The model under review builds one solid part; all positions refer to its coordinate system, in mm. Face numbers are marked on the shaded views. A direction names the side the tool comes from. Coordinates: 2 decimals unless noted, no trailing zeros. Order: outer loops, then holes, each group sorted by start corner. A loop starts at its lowest first (then second) coordinate and runs counter-clockwise, first axis right, second up. Notation, with made-up numbers: M -16,87.5 L 23,87.5 A29 cw 23,125.5 Z; hole C -5,46 d5. An arc over 180 degrees is marked long. One line per item, written item: value.
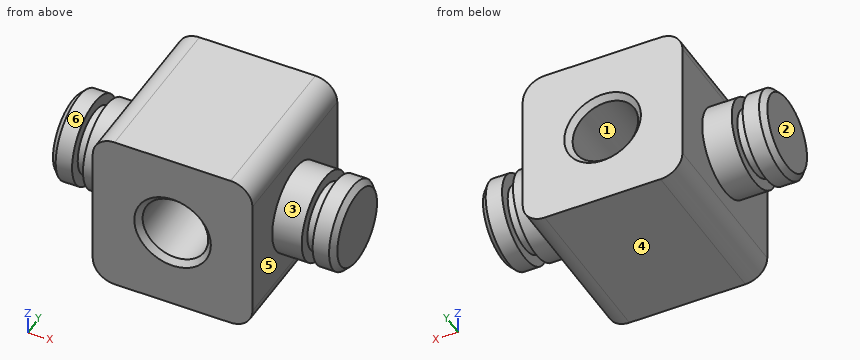
```python
from build123d import *

# Parameters (mm, degrees)
F2_DEPTH  = 381
F3_R      = 101.6
F4_DEPTH  = 68.58
F5_R      = 101.6
F6_DEPTH  = 68.58
F7_R      = 76.2
F8_DEPTH  = 508
F9_SIZE2  = 12.7
F9_SIZE   = 12.7
F11_R     = 76.2
F12_DEPTH = 25.4
F10_R     = 76.2
F13_DEPTH = 25.4
F14_R     = 101.6
F14_R_2   = 76.2
F15_DEPTH = 50.8
F16_R     = 101.6
F17_DEPTH = 50.8
F18_SIZE2 = 12.7
F18_SIZE  = 12.7


with BuildPart() as f2:
    # F1 (on Front) → F2 (new body)
    with BuildSketch(Plane.XZ):
        with BuildLine():
            ThreePointArc((-185.42, -139.7), (-170.541024, -175.621024), (-134.62, -190.5))
            Line((-134.62, -190.5), (134.62, -190.5))
            ThreePointArc((134.62, -190.5), (170.541024, -175.621024), (185.42, -139.7))
            Line((185.42, -139.7), (185.42, 139.7))
            ThreePointArc((185.42, 139.7), (170.541024, 175.621024), (134.62, 190.5))
            Line((134.62, 190.5), (-134.62, 190.5))
            ThreePointArc((-134.62, 190.5), (-170.541024, 175.621024), (-185.42, 139.7))
            Line((-185.42, 139.7), (-185.42, -139.7))
        make_face()
    extrude(amount=F2_DEPTH)

    # F3 (on face) → F4 (join)
    with BuildSketch(Plane.YZ.offset(185.42)):
        with Locations((-190.5, 0)):
            Circle(F3_R)
    extrude(amount=F4_DEPTH)

    # F5 (on face) → F6 (join)
    with BuildSketch(Plane(origin=(-185.42, 0, 0), x_dir=(0, -1, 0), z_dir=(-1, 0, 0))):
        with Locations((190.5, 0)):
            Circle(F5_R)
    extrude(amount=F6_DEPTH)

    # F7 (on face) → F8 (cut)
    with BuildSketch(Plane.XZ.offset(381)):
        Circle(F7_R)
    extrude(amount=-F8_DEPTH, mode=Mode.SUBTRACT)

    # F9
    f9_edges = [f2.edges().sort_by_distance(p)[0] for p in [
        (-76.2, -381, 0),
        (-76.2, 0, 0),
    ]]
    chamfer(f9_edges, length=F9_SIZE, length2=F9_SIZE2)

    # F11 (on face) → F12 (join)
    with BuildSketch(Plane.YZ.offset(254)):
        with Locations((-190.5, 0)):
            Circle(F11_R)
    extrude(amount=F12_DEPTH)

    # F10 (on face) → F13 (join)
    with BuildSketch(Plane(origin=(-254, 0, 0), x_dir=(0, -1, 0), z_dir=(-1, 0, 0))):
        with Locations((190.5, 0)):
            Circle(F10_R)
    extrude(amount=F13_DEPTH)

    # F14 (on face) → F15 (join)
    with BuildSketch(Plane.YZ.offset(279.4)):
        with Locations((-190.5, 0)):
            Circle(F14_R)
        with Locations((-190.5, 0)):
            Circle(F14_R_2, mode=Mode.SUBTRACT)
        with Locations((-190.5, 0)):
            Circle(F14_R)
        with Locations((-190.5, 0)):
            Circle(F14_R_2)
    extrude(amount=F15_DEPTH)

    # F16 (on face) → F17 (join)
    with BuildSketch(Plane(origin=(-279.4, 0, 0), x_dir=(0, -1, 0), z_dir=(-1, 0, 0))):
        with Locations((190.5, 0)):
            Circle(F16_R)
    extrude(amount=F17_DEPTH)

    # F18
    f18_edges = [f2.edges().sort_by_distance(p)[0] for p in [
        (330.2, -292.1, 0),
        (-330.2, -88.9, 0),
    ]]
    chamfer(f18_edges, length=F18_SIZE, length2=F18_SIZE2)


solid = f2.part
```
(1) We need section A-A, the plane x = 0. State the section outline as (y, z) points.
Geometry results:
outline: M -381,-190.5 L 0,-190.5 L 0,-88.9 L -12.7,-76.2 L -368.3,-76.2 L -381,-88.9 Z; M -381,88.9 L -368.3,76.2 L -12.7,76.2 L 0,88.9 L 0,190.5 L -381,190.5 Z
(2) For L1, parallel to Z at x = 0, y = -194.5; L2, parallel to X at y = -163, z = -76.5; L3, parallel to X at y = -236.5, z = 67, list the stretches that pass through material, from the lowest coordinate up.
Geometry results:
L1: z = -190.5 to -76.2, 76.2 to 190.5
L2: x = -330.2 to -279.4, -254 to 254, 279.4 to 330.2
L3: x = -330.2 to -279.4, -254 to -36.3, 36.3 to 254, 279.4 to 330.2
(3) Insertion check: pin 1 Ø3 at (y, z) = (-205.5, -114.5) entering from -X; pin 2 Ø8 at (y, z) = (-130.5, 72.5) entering from +X. Each pin has a flat end and moves straight along its axis. Give the tip position at first contact, or say it passes through.
Geometry results:
pin 1: stops at x = -185.42
pin 2: stops at x = 328.99
(4) We need section B-B, the plane z = 158.5. State the section outline as (x, y) points, plus the area to 3 significant figures.
Geometry results:
outline: M -181.81,-381 L 181.81,-381 L 181.81,0 L -181.81,0 Z
area: 139,000 mm2
(5) Mouldability with a two-part tool opening along X and no side actions: class the marked faces 1, 2 and 3 as +X half, -X half, draft (parallel to the pull), parting line (faces both ways), or undercut.
Geometry results:
face 1: undercut
face 2: -X half
face 3: draft
(6) Tool access review of the marked faces 4, 5 and 6: name each direction out of +Z, -Z, +X, -X, +Y, -Y from which nothing blocks a thin tool from reaching the whole face with its end or side.
Geometry results:
face 4: -Z, +X, -X, +Y, -Y
face 5: +X
face 6: -X
